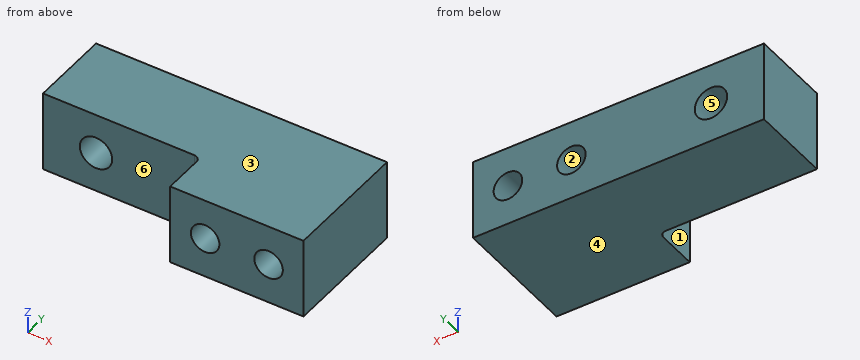
from build123d import *

# Parameters (mm, degrees)
BOSS_EXTRUDE1_DEPTH         = 12.7
M4_CLEARANCE_HOLE1_D        = 4.5
TAP_DRILL_FOR_1_4_20_TAP1_D = 5.1054


with BuildPart() as part:
    # Sketch1 → Boss-Extrude1 (new body)
    with BuildSketch(Plane.XY):
        with BuildLine():
            Line((0, 0), (21, 0))
            Line((21, 0), (21, 20))
            Line((21, 20), (-24.85, 20))
            Line((-24.85, 20), (-24.85, 7.3))
            Line((-24.85, 7.3), (-1, 7.3))
            ThreePointArc((-1, 7.3), (-0.292893219, 7.007106781), (0, 6.3))
            Line((0, 6.3), (0, 0))
        make_face()
    extrude(amount=BOSS_EXTRUDE1_DEPTH)

    # M4 Clearance Hole1 (through all)
    with Locations(Plane(origin=(0, 20, 0), x_dir=(1, 0, 0), z_dir=(0, 1, 0))):
        with Locations((5.5, -6.35), (15.5, -6.35)):
            Hole(M4_CLEARANCE_HOLE1_D / 2)

    # Tap Drill for 1/4-20 Tap1 (through all)
    with Locations(Plane(origin=(0, 20, 0), x_dir=(1, 0, 0), z_dir=(0, 1, 0))):
        with Locations((-16.5, -6.35)):
            Hole(TAP_DRILL_FOR_1_4_20_TAP1_D / 2)


solid = part.part
Geometry check sheet. Reference: the model listing, model coordinates, mm. Face numbers are marked on the shaded views. A direction names the side the tool comes from. Give positions to 0.01 mm unless a question says otherwise; leave off trailing zeros. Loops run counter-clockwise (first coordinate to the right, second up) from the corner with the lowest first, then second, coordinate; pieces in that order, holes last. Notation, with made-up numbers: (-38, 3) -> (-9, 3) arc R21 ccw to (-9, 21) -> close; hole circle Ø2 at (60, 48). An arc over 180 degrees is marked (long way). Answer in a Markdown table with one row per item. Add a question column.
1) Cross-section at C-C on y = 18. Record the boundary of the cut face in (x, z).
2) Material ranges on probe 1 along Z at (x, y) = (-16.5, 17); probe 2 along Z at (x, y) = (5.5, 13.5); probe 3 along X at (y, z) = (1.75, 10.25), recorded low to high. Write a range as from..to.
3) Set-up check for the marked faces 5 and 6: record each of +Z, -Z, +X, -X, +Y, -Y from which the full face is reachable in a straight line by a thin tool's end or side.
4) Cross-section at D-D on z = 1.5. Record the boundary of the cut face in (x, y), and give its area (3 significant figures).
5) Cross-section at A-A on x = -16.5. Record the boundary of the cut face in (y, z).
6) Cross-section at B-B on z = 6.35. Record the boundary of the cut face in (x, y), and give its area (3 significant figures).
7) Draft check along Z on the marked faces 1, 2, 3 and 4. Enter one of: pulls with the +Z half, pulls with the -Z half, needs draft (parallel to the pull), parting line crosses it, or undercut.
8) Gauge pin test, flat ends, axial feed: P1, Ø5, axis at y = 4.5, z = 4, coming from the -X side; P2, Ø4, axis at x = -17.5, z = 6.5, coming from the -Y side; P3, Ø1.5, axis at y = 6, z = 11, coming from the -X side. Record the tip position at first contact, or that the pin passes through.
Outcome:
| question | item | result |
|---|---|---|
| 1 | outline | (-24.85, 0) -> (21, 0) -> (21, 12.7) -> (-24.85, 12.7) -> close; hole circle Ø5.11 at (-16.5, 6.35); hole circle Ø4.5 at (5.5, 6.35); hole circle Ø4.5 at (15.5, 6.35) |
| 2 | probe 1 | z = 0..3.8, 8.9..12.7 |
| 2 | probe 2 | z = 0..4.1, 8.6..12.7 |
| 2 | probe 3 | x = 0..21 |
| 3 | face 5 | +Y, -Y |
| 3 | face 6 | +Z, -Z, -X, -Y |
| 4 | outline | (-24.85, 7.3) -> (-1, 7.3) arc R1 cw to (0, 6.3) -> (0, 0) -> (21, 0) -> (21, 20) -> (-24.85, 20) -> close |
| 4 | area | 736 mm^2 |
| 5 | outline | (7.3, 0) -> (20, 0) -> (20, 3.8) -> (7.3, 3.8) -> close; (7.3, 8.9) -> (20, 8.9) -> (20, 12.7) -> (7.3, 12.7) -> close |
| 6 | outline | (-24.85, 7.3) -> (-19.05, 7.3) -> (-19.05, 20) -> (-24.85, 20) -> close; (-13.95, 7.3) -> (-1, 7.3) arc R1 cw to (0, 6.3) -> (0, 0) -> (3.25, 0) -> (3.25, 20) -> (-13.95, 20) -> close; (7.75, 0) -> (13.25, 0) -> (13.25, 20) -> (7.75, 20) -> close; (17.75, 0) -> (21, 0) -> (21, 20) -> (17.75, 20) -> close |
| 6 | area | 491 mm^2 |
| 7 | face 1 | needs draft |
| 7 | face 2 | undercut |
| 7 | face 3 | pulls with the +Z half |
| 7 | face 4 | pulls with the -Z half |
| 8 | P1 | stops at x = -0.29 |
| 8 | P2 | stops at y = 7.3 |
| 8 | P3 | stops at x = -0.11 |
